Check sheet for the modelled part. Datum: model origin and axes. Units: mm. Face numbers are marked on the shaded views. A direction names the side the tool comes from. Round coordinates to 2 decimals unless told otherwise and drop trailing zeros. Order: outer loops, then holes, each group sorted by start corner. A loop starts at its lowest first (then second) coordinate and runs counter-clockwise, first axis right, second up. Notation, with made-up numbers: (27, -25.75) -> (75, -25.75) arc R33 cw to (75, 3.25) -> close; hole circle Ø9 at (29, -35.75). An arc over 180 degrees is marked (long way). Answer in a Markdown table with one row per item.
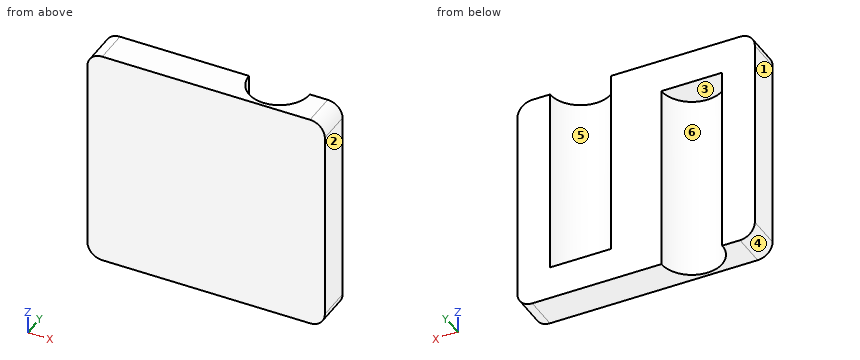
```python
from build123d import *

# Parameters (mm, degrees)
SKETCH1_W           = 32
SKETCH1_H           = 6.5
BOSS_EXTRUDE1_DEPTH = 30
FILLET1_R           = 2
SKETCH2_R           = 4.1
CUT_EXTRUDE1_DEPTH  = 25.5
SKETCH3_R           = 4.1
CUT_EXTRUDE2_DEPTH  = 25.5
SKETCH5_W           = 32
SKETCH5_H           = 0.1
CUT_EXTRUDE3_DEPTH  = 37.629308734
SKETCH6_W           = 32
SKETCH6_H           = 1.8
CUT_EXTRUDE4_DEPTH  = 37.629308734


with BuildPart() as part:
    # Sketch1 → Boss-Extrude1 (new body)
    with BuildSketch(Plane.XY):
        with Locations((3.954315745, -3.347843701)):
            Rectangle(SKETCH1_W, SKETCH1_H)
    extrude(amount=BOSS_EXTRUDE1_DEPTH)

    # Fillet1
    fillet1_edges = [part.edges().sort_by_distance(p)[0] for p in [
        (19.954315745, -3.347843701, 30),
        (-12.045684255, -3.347843701, 30),
        (19.954315745, -3.347843701, 0),
        (-12.045684255, -3.347843701, 0),
    ]]
    fillet(fillet1_edges, radius=FILLET1_R)

    # Sketch2 → Cut-Extrude1 (cut)
    with BuildSketch(Plane(origin=(0, 0, 0), x_dir=(-1, 0, 0), z_dir=(0, 0, -1))):
        with Locations((3.545684255, -0.197843701)):
            Circle(SKETCH2_R)
    extrude(amount=-CUT_EXTRUDE1_DEPTH, mode=Mode.SUBTRACT)

    # Sketch3 → Cut-Extrude2 (cut)
    with BuildSketch(Plane.XY.offset(30)):
        with Locations((11.454315745, -0.197843701)):
            Circle(SKETCH3_R)
    extrude(amount=-CUT_EXTRUDE2_DEPTH, mode=Mode.SUBTRACT)

    # Sketch5 → Cut-Extrude3 (cut, through all)
    with BuildSketch(Plane.XY.offset(30)):
        with Locations((3.954315745, -0.147843701)):
            Rectangle(SKETCH5_W, SKETCH5_H)
    extrude(amount=-CUT_EXTRUDE3_DEPTH, mode=Mode.SUBTRACT)

    # Sketch6 → Cut-Extrude4 (cut, through all)
    with BuildSketch(Plane.XY.offset(30)):
        with Locations((3.954315745, -5.697843701)):
            Rectangle(SKETCH6_W, SKETCH6_H)
    extrude(amount=-CUT_EXTRUDE4_DEPTH, mode=Mode.SUBTRACT)


solid = part.part
```
(1) Section check C-C on x = -2.5. Record the boundary of the cut face in (y, z), plus the area to 3 significant figures.
Solutions:
| item | result |
|---|---|
| outline | (-4.8, 0) -> (-4.16, 0) -> (-4.16, 25.5) -> (-0.2, 25.5) -> (-0.2, 30) -> (-4.8, 30) -> close |
| area | 36.9 mm^2 |
(2) Tool access check on the marked faces 4, 5 and 6. Record the directions out of +Z, -Z, +X, -X, +Y, -Y that give a thin tool (end or side, any length) a straight path to the whole face; none if there is none.
Solutions:
| item | result |
|---|---|
| face 4 | -Z, -X, +Y, -Y |
| face 5 | +Z, +Y |
| face 6 | -Z, +Y |
(3) Draft check along X on the marked faces 1, 2 and 3. Enter one of: pulls with the +X half, pulls with the -X half, needs draft (parallel to the pull), parting line crosses it, or undercut.
Solutions:
| item | result |
|---|---|
| face 1 | pulls with the -X half |
| face 2 | pulls with the +X half |
| face 3 | undercut |
(4) Section check A-A on y = -1.85. Record the boundary of the cut face in (x, z).
Solutions:
| item | result |
|---|---|
| outline | (-12.05, 2) arc R2 ccw to (-10.05, 0) -> (-7.3, 0) -> (-7.3, 25.5) -> (0.21, 25.5) -> (0.21, 0) -> (17.95, 0) arc R2 ccw to (19.95, 2) -> (19.95, 28) arc R2 ccw to (17.95, 30) -> (15.21, 30) -> (15.21, 4.5) -> (7.7, 4.5) -> (7.7, 30) -> (-10.05, 30) arc R2 ccw to (-12.05, 28) -> close |
(5) Scan lines: probe 1 along X at (y, z) = (-2.05, 14.25); probe 2 along X at (y, z) = (-2.2, 14); probe 3 along Z at (x, y) = (11, -3.65). Record each from-to range of solid material in increasing order. Write a range as from..to.
Solutions:
| item | result |
|---|---|
| probe 1 | -12.05..-7.2, 0.11..7.8, 15.11..19.95 |
| probe 2 | -12.05..-7.12, 0.03..7.88, 15.03..19.95 |
| probe 3 | 0..4.5 |
(6) Depth check by flat-ended pin: pin 1 Ø1.2 at (x, y) = (10.5, -1.5) entering from +Z. Enter the tip coordinate at first touch or a pass-through.
Solutions:
| item | result |
|---|---|
| pin 1 | z = 4.5 |
(7) Section check B-B on z = 19.75. Record the boundary of the cut face in (x, y), plus the area to 3 significant figures.
Solutions:
| item | result |
|---|---|
| outline | (-12.05, -4.8) -> (19.95, -4.8) -> (19.95, -0.2) -> (15.55, -0.2) arc R4.1 cw to (7.35, -0.2) -> (0.55, -0.2) arc R4.1 cw to (-7.65, -0.2) -> (-12.05, -0.2) -> close |
| area | 94.4 mm^2 |
(8) Section check D-D on z = 27.25. Record the boundary of the cut face in (x, y).
Solutions:
| item | result |
|---|---|
| outline | (-12.05, -4.8) -> (19.95, -4.8) -> (19.95, -0.2) -> (15.55, -0.2) arc R4.1 cw to (7.35, -0.2) -> (-12.05, -0.2) -> close |
